Can you work these out from the model? Positions are in its coordinate system, mm. Coordinates: 2 decimals unless noted, no trailing zeros. Order: outer loops, then holes, each group sorted by start corner. A loop starts at its lowest first (then second) coordinate and runs counter-clockwise, first axis right, second up. Notation, with made-up numbers: (24.25, 79) -> (34.25, 79) arc R16 ccw to (34.25, 98) -> close; hole circle Ø3 at (23, -29.5). An arc over 180 degrees is marked (long way). Answer in a Markdown table with one row per item.
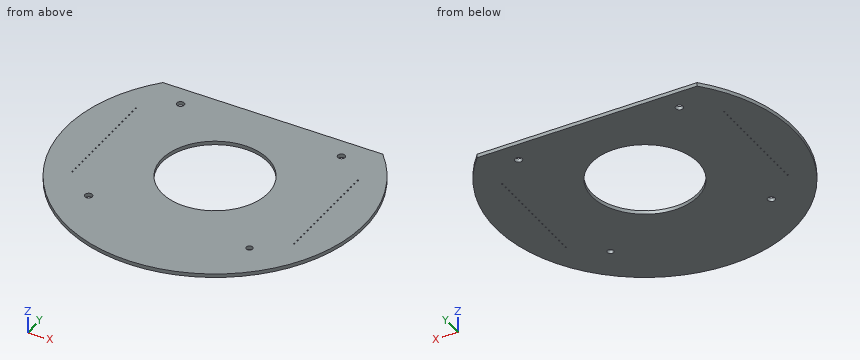
```python
from build123d import *

# Parameters (mm, degrees)
SKETCH1_R           = 65
BOSS_EXTRUDE1_DEPTH = 1.6
SKETCH3_R           = 0.3
CUT_EXTRUDE1_DEPTH  = 1.6
SKETCH4_W           = 100
SKETCH4_H           = 26
CUT_EXTRUDE2_DEPTH  = 10
SKETCH5_R           = 1.6
SKETCH5_R_2         = 1.36
CUT_EXTRUDE3_DEPTH  = 10
SKETCH6_R           = 23.1
CUT_EXTRUDE4_DEPTH  = 1.6


with BuildPart() as part:
    # Sketch1 → Boss-Extrude1 (new body)
    with BuildSketch(Plane.XY):
        Circle(SKETCH1_R)
    extrude(amount=BOSS_EXTRUDE1_DEPTH)

    # Sketch3 → Cut-Extrude1 (cut)
    with BuildSketch(Plane.XY.offset(1.6)):
        with Locations((48.26, -24.130008683)):
            Circle(SKETCH3_R)
        with Locations((-48.26, -24.130008683)):
            Circle(SKETCH3_R)
        with Locations((-48.26, -21.590008683)):
            Circle(SKETCH3_R)
        with Locations((48.26, -21.590008683)):
            Circle(SKETCH3_R)
        with Locations((-48.26, -19.050008683)):
            Circle(SKETCH3_R)
        with Locations((48.26, -19.050008683)):
            Circle(SKETCH3_R)
        with Locations((-48.26, -16.510008683)):
            Circle(SKETCH3_R)
        with Locations((48.26, -16.510008683)):
            Circle(SKETCH3_R)
        with Locations((-48.26, -13.970008683)):
            Circle(SKETCH3_R)
        with Locations((48.26, -13.970008683)):
            Circle(SKETCH3_R)
        with Locations((-48.26, -11.430008683)):
            Circle(SKETCH3_R)
        with Locations((48.26, -11.430008683)):
            Circle(SKETCH3_R)
        with Locations((-48.26, -8.890008683)):
            Circle(SKETCH3_R)
        with Locations((48.26, -8.890008683)):
            Circle(SKETCH3_R)
        with Locations((-48.26, -6.350008683)):
            Circle(SKETCH3_R)
        with Locations((48.26, -6.350008683)):
            Circle(SKETCH3_R)
        with Locations((-48.26, -3.810008683)):
            Circle(SKETCH3_R)
        with Locations((48.26, -3.810008683)):
            Circle(SKETCH3_R)
        with Locations((-48.26, -1.270008683)):
            Circle(SKETCH3_R)
        with Locations((48.26, -1.270008683)):
            Circle(SKETCH3_R)
        with Locations((-48.26, 1.269991317)):
            Circle(SKETCH3_R)
        with Locations((48.26, 1.269991317)):
            Circle(SKETCH3_R)
        with Locations((-48.26, 3.809991317)):
            Circle(SKETCH3_R)
        with Locations((48.26, 3.809991317)):
            Circle(SKETCH3_R)
        with Locations((-48.26, 6.349991317)):
            Circle(SKETCH3_R)
        with Locations((48.26, 6.349991317)):
            Circle(SKETCH3_R)
        with Locations((-48.26, 8.889991317)):
            Circle(SKETCH3_R)
        with Locations((48.26, 8.889991317)):
            Circle(SKETCH3_R)
        with Locations((-48.26, 11.429991317)):
            Circle(SKETCH3_R)
        with Locations((48.26, 11.429991317)):
            Circle(SKETCH3_R)
        with Locations((-48.26, 13.969991317)):
            Circle(SKETCH3_R)
        with Locations((48.26, 13.969991317)):
            Circle(SKETCH3_R)
        with Locations((-48.26, 16.509991317)):
            Circle(SKETCH3_R)
        with Locations((48.26, 16.509991317)):
            Circle(SKETCH3_R)
        with Locations((-48.26, 19.049991317)):
            Circle(SKETCH3_R)
        with Locations((48.26, 19.049991317)):
            Circle(SKETCH3_R)
        with Locations((-48.26, 21.589991317)):
            Circle(SKETCH3_R)
        with Locations((48.26, 21.589991317)):
            Circle(SKETCH3_R)
        with Locations((-48.26, 24.129991317)):
            Circle(SKETCH3_R)
        with Locations((48.26, 24.129991317)):
            Circle(SKETCH3_R)
    extrude(amount=-CUT_EXTRUDE1_DEPTH, mode=Mode.SUBTRACT)

    # Sketch4 → Cut-Extrude2 (cut)
    with BuildSketch(Plane.XY.offset(1.6)):
        with Locations((0, 57)):
            Rectangle(SKETCH4_W, SKETCH4_H)
    extrude(amount=-CUT_EXTRUDE2_DEPTH, mode=Mode.SUBTRACT)

    # Sketch5 → Cut-Extrude3 (cut)
    with BuildSketch(Plane.XY.offset(1.6)):
        with Locations((-35, 35)):
            Circle(SKETCH5_R)
        with Locations((35, 35)):
            Circle(SKETCH5_R)
        with Locations((-35, -35)):
            Circle(SKETCH5_R)
        with Locations((35, -35)):
            Circle(SKETCH5_R_2)
    extrude(amount=-CUT_EXTRUDE3_DEPTH, mode=Mode.SUBTRACT)

    # Sketch6 → Cut-Extrude4 (cut)
    with BuildSketch(Plane.XY.offset(1.6)):
        Circle(SKETCH6_R)
    extrude(amount=-CUT_EXTRUDE4_DEPTH, mode=Mode.SUBTRACT)


solid = part.part
```
(1) Suppose I cut it at C-C (y = 35). Please give me the cut outline in (x, z).
Response values:
| item | result |
|---|---|
| outline | (-54.77, 0) -> (-36.6, 0) -> (-36.6, 1.6) -> (-54.77, 1.6) -> close; (-33.4, 0) -> (33.4, 0) -> (33.4, 1.6) -> (-33.4, 1.6) -> close; (36.6, 0) -> (54.77, 0) -> (54.77, 1.6) -> (36.6, 1.6) -> close |
(2) Suppose I cut it at B-B (x = -35). Please give me the cut outline in (y, z).
Response values:
| item | result |
|---|---|
| outline | (-54.77, 0) -> (-36.6, 0) -> (-36.6, 1.6) -> (-54.77, 1.6) -> close; (-33.4, 0) -> (33.4, 0) -> (33.4, 1.6) -> (-33.4, 1.6) -> close; (36.6, 0) -> (44, 0) -> (44, 1.6) -> (36.6, 1.6) -> close |
(3) Suppose I cut it at D-D (z = 0.65). Count the separate pieces of the cut face and the enclosed holes in it, and give its area (3 significant figures).
Response values:
| item | result |
|---|---|
| separate pieces | 1 |
| enclosed holes | 45 |
| area | 10,200 mm2 |
(4) I need wall thicknesses on line 1 (X direction, y = 11.5, z = 1.15); line 2 (Y direction, x = 0, z = 0.45); line 3 (X direction, y = -3, z = 1.15). Which ranges of each line are inside material? Lowest first, please. Write a range as [from, to].
Response values:
| item | result |
|---|---|
| line 1 | [-63.97, -48.55], [-47.97, -20.03], [20.03, 47.97], [48.55, 63.97] |
| line 2 | [-65, -23.1], [23.1, 44] |
| line 3 | [-64.93, -22.9], [22.9, 64.93] |
(5) Will these pins go through, and if not, where does the flat tip stop? pin 1 Ø8 at (x, y) = (-40, 25) entering from -Z; pin 2 Ø8 at (x, y) = (0, 18) entering from -Z.
Response values:
| item | result |
|---|---|
| pin 1 | z = 0 |
| pin 2 | through |
(6) Suppose I cut it at A-A (x = 0). Please give me the cut outline in (y, z).
Response values:
| item | result |
|---|---|
| outline | (-65, 0) -> (-23.1, 0) -> (-23.1, 1.6) -> (-65, 1.6) -> close; (23.1, 0) -> (44, 0) -> (44, 1.6) -> (23.1, 1.6) -> close |
